from build123d import *

# Parameters (mm, degrees)
SKETCH1_W           = 32
SKETCH1_H           = 114
BOSS_EXTRUDE1_DEPTH = 96
CUT_EXTRUDE1_REACH  = 157.637
CUT_EXTRUDE2_REACH  = 152.756
SKETCH8_R           = 19
BOSS_EXTRUDE2_DEPTH = 52


with BuildPart() as part:
    # Sketch1 → Boss-Extrude1 (new body)
    with BuildSketch(Plane.XY):
        with Locations((-16, 57)):
            Rectangle(SKETCH1_W, SKETCH1_H)
    extrude(amount=-BOSS_EXTRUDE1_DEPTH)

    # Sketch4 → Cut-Extrude1 (cut, up to next)
    with BuildSketch(Plane(origin=(-18.160548949, -5.315282619, 2.270068619), x_dir=(0.11431729078371765, 0.033458719253771, 0.9928806933029609), z_dir=(-0.9529047420591578, -0.27889894889536315, 0.11911309275739475)), mode=Mode.PRIVATE) as cut_extrude1_sk1:
        Polygon((-98.974699862, 8.988760105), (-2.286345816, 48.337993792), (-2.286345816, 5.617975065), align=None)
    cut_extrude1_tool1 = extrude(cut_extrude1_sk1.sketch, amount=CUT_EXTRUDE1_REACH, mode=Mode.PRIVATE) & part.part
    add(cut_extrude1_tool1.solids().sort_by_distance((-28, 13.666667, -32))[0], mode=Mode.SUBTRACT)

    # Sketch3 → Cut-Extrude2 (cut, up to next)
    with BuildSketch(Plane(origin=(-48.457659878, 14.18272972, 6.057207485), x_dir=(0.11431729078371765, -0.033458719253771, 0.9928806933029609), z_dir=(-0.9529047420591578, 0.27889894889536315, 0.11911309275739475)), mode=Mode.PRIVATE) as cut_extrude2_sk1:
        Polygon((-6.100639811, 61.072070607), (-6.100639811, 103.792089334), (-102.788993857, 100.421304294), align=None)
    cut_extrude2_tool1 = extrude(cut_extrude2_sk1.sketch, amount=CUT_EXTRUDE2_REACH, mode=Mode.PRIVATE) & part.part
    add(cut_extrude2_tool1.solids().sort_by_distance((-28, 100.333333, -32))[0], mode=Mode.SUBTRACT)

    # Sketch8 → Boss-Extrude2 (add)
    with BuildSketch(Plane(origin=(0, 0, 0), x_dir=(0, 0, -1), z_dir=(1, 0, 0))):
        with BuildLine():
            Line((96, 114), (149.250761153, 85.132086383))
            ThreePointArc((149.250761153, 85.132086383), (166, 57), (149.250761153, 28.867913617))
            Line((149.250761153, 28.867913617), (96, 0))
            Line((96, 0), (96, 114))
        make_face()
        with Locations((134, 57)):
            Circle(SKETCH8_R, mode=Mode.SUBTRACT)
    extrude(amount=-BOSS_EXTRUDE2_DEPTH)


solid = part.part
For this review, take the finished solid that the model builds, in its own axes (mm). A direction names the side the tool comes from. Give positions to 0.01 mm unless a question says otherwise; leave off trailing zeros. Order: outer loops, then holes, each group sorted by start corner. A loop starts at its lowest first (then second) coordinate and runs counter-clockwise, first axis right, second up. Notation, with made-up numbers: (26.25, 89) - (48.25, 89) arc R17 ccw to (48.25, 120) - close; hole circle Ø10 at (53.25, -7.5). An arc over 180 degrees is marked (long way). Answer as a JSON object with one key per item and string values. Group by question number.
Item 1: Machinability: for faces 5 (the flat face through (-13, 58, 0)), 6 (the flat face through (-32, 56, -58)), which of the approach directions +Z, -Z, +X, -X, +Y, -Y give a long, thin tool a straight path to every point of the face, cutting with its end or side? Answer none if there is none.
Item 2: Take a section at C-C on z = -134. Give the boundary of the cut face in (x, y).
Item 3: Clearance check with flat-ended pins moving along their axes: pin 1 Ø2 at (x, z) = (-36, -128.5) entering from -Y; pin 2 Ø5 at (y, z) = (64, -55.5) entering from +X; pin 3 Ø2 at (y, z) = (22.5, -57) entering from -X; pin 4 Ø1.5 at (x, y) = (-20, 63) entering from -Z. State where each tip first meets the part, or that it passes through.
Item 4: Take a section at D-D on y = 31. Give the boundary of the cut face in (x, z), and give its area (3 significant figures).
Item 5: Draft analysis for pull direction Y (two halves, no side actions). For faces 1 (the flat face through (-52, 45, -116)), 2 (the cylindrical face through (-25.64, 62.71, -152.12)), 3 (the flat face through (-27.73, 99.26, -27.34)), 4 (the cylindrical face through (-26, 57, -166)), state which applies: pulls with the +Y half, pulls with the -Y half, needs draft (parallel to the pull), parting line crosses it, or undercut.
Item 6: Take a section at B-B on x = -23. Give the boundary of the cut face in (y, z).
Item 7: Wall thickness on line 1 along X through (y, z) = (47.5, -69); line 2 along Z through (x, y) = (-14.5, 60); line 3 along Y through (x, z) = (-21.5, -125): over which ranges is each line inside the solid? List them lowest first.
Item 8: Take a section at A-A on y = 57. Give the boundary of the cut face in (x, z), and give its area (3 significant figures).
Reported:
{
 "1": {"face 5": "+Z, +X, -X, +Y, -Y", "face 6": "+Z, -X, +Y, -Y"},
 "2": {"outline": "(-52, 20.6) - (0, 20.6) - (0, 38) - (-52, 38) - close; (-52, 76) - (0, 76) - (0, 93.4) - (-52, 93.4) - close"},
 "3": {"pin 1": "y = 17.08", "pin 2": "x = 0", "pin 3": "x = -32", "pin 4": "z = -165.57"},
 "4": {"outline": "(-52, -152.65) - (0, -152.65) - (0, 0) - (-29.07, 0) - (-32, -23.41) - (-32, -96) - (-52, -96) - close", "area": "5,980 mm^2"},
 "5": {"face 1": "needs draft", "face 2": "undercut", "face 3": "pulls with the +Y half", "face 4": "parting line crosses it"},
 "6": {"outline": "(0, -96) - (28.87, -149.25) arc R32 ccw to (85.13, -149.25) - (114, -96) - (114, -24) - (103.75, 0) - (10.25, 0) - (0, -24) - close; hole circle Ø38 at (57, -134)"},
 "7": {"line 1": "-32 to 0", "line 2": "-165.86 to -152.76, -115.24 to 0", "line 3": "15.72 to 40.27, 73.73 to 98.28"},
 "8": {"outline": "(-52, -166) - (0, -166) - (0, -153) - (-52, -153) - close; (-52, -115) - (0, -115) - (0, 0) - (-32, 0) - (-32, -96) - (-52, -96) - close", "area": "4,740 mm^2"}
}
